For this review, take the finished solid that the model builds, in its own axes (mm). Face numbers are marked on the shaded views. A direction names the side the tool comes from. Coordinates: 2 decimals unless noted, no trailing zeros. Loops run counter-clockwise (first coordinate to the right, second up) from the corner with the lowest first, then second, coordinate; pieces in that order, holes last. Notation, with made-up numbers: (-13, 15) - (15, 15) arc R18 cw to (15, 45) - close; hole circle Ø7 at (31, 40). An arc over 180 degrees is marked (long way). One line per item, written item: value. Start each with the question number.
1. Take a section at A-A, the plane z = 10.75. State the section outline as (x, y) points, and give its area (3 significant figures).
2. To check wall thickness, follow line 1 (X direction, y = -37.5, z = 8.5); line 2 (Y direction, x = -3.5, z = 9.5); line 3 (Z direction, x = 22.5, y = -36). State the ranges of each line that lie inside material, in increasing order. Write a range as from..to.
3. Insertion check: pin 1 (6.5 mm diameter, centred on x = 11.5, y = -7.5, fed in from +Z); pin 2 (2.5 mm diameter, centred on x = -23.3, y = -35.37, fed in from +Z); pin 3 (2 mm diameter, centred on x = 16.5, z = 4.5, fed in from +Y). Each pin has a flat end and moves straight along its axis. Give the tip position at first contact, or say it passes through.
4. Take a section at B-B, the plane x = 4. State the section outline as (y, z) points.
5. Take a section at C-C, the plane y = -33. State the section outline as (x, z) points, and give its area (3 significant figures).
6. For the marked faces 1 and 2, list the 3-axis set-ups (+Z, -Z, +X, -X, +Y, -Y) from which the entire face can be reached by the end or side of a thin tool; tool diameter is ignored.
```python
from build123d import *

# Parameters (mm, degrees)
F0_W     = 65
F0_H     = 15
F0_R     = 2.85
F1_DEPTH = 12
F2_W     = 65
F2_H     = 13
F3_DEPTH = 8.8
F4_R     = 1.2
F5_R     = 1.05
F6_DEPTH = 15
F8_DEPTH = 6.9


with BuildPart() as f1:
    # F0 (on Top) → F1 (new body)
    with BuildSketch(Plane.XY):
        with Locations((0.397058, -10.369431)):
            Rectangle(F0_W, F0_H)
        with Locations((-20.602942, -9.369431)):
            Circle(F0_R, mode=Mode.SUBTRACT)
        with Locations((21.397058, -9.369431)):
            Circle(F0_R, mode=Mode.SUBTRACT)
        with BuildLine():
            Line((32.897058, -17.869431), (-32.102942, -17.869431))
            Line((-32.102942, -17.869431), (-32.102942, -35.869431))
            ThreePointArc((-32.102942, -35.869431), (-25.659291, -51.42578), (-10.102942, -57.869431))
            Line((-10.102942, -57.869431), (10.897058, -57.869431))
            ThreePointArc((10.897058, -57.869431), (26.453407, -51.42578), (32.897058, -35.869431))
            Line((32.897058, -35.869431), (32.897058, -17.869431))
        make_face()
    extrude(amount=F1_DEPTH)

    # F2 (on face) → F3 (cut)
    with BuildSketch(Plane.XY.offset(12)):
        with Locations((0.397058, -9.369431)):
            Rectangle(F2_W, F2_H)
    extrude(amount=-F3_DEPTH, mode=Mode.SUBTRACT)

    # F4
    f4_edges = [f1.edges().sort_by_distance(p)[0] for p in [
        (-32.102942, -19.369431, 0),
        (0.397058, -57.869431, 0),
        (32.897058, -19.369431, 0),
    ]]
    fillet(f4_edges, radius=F4_R)

    # F5 (on face) → F6 (cut)
    with BuildSketch(Plane(origin=(0, 0, 0), x_dir=(1, 0, 0), z_dir=(0, 0, -1))):
        with Locations((23.697058, 35.369431)):
            Circle(F5_R)
        with Locations((-23.302942, 35.369431)):
            Circle(F5_R)
    extrude(amount=-F6_DEPTH, mode=Mode.SUBTRACT)

    # F7 (on face) → F8 (cut)
    with BuildSketch(Plane.XY.offset(12)):
        Polygon((25.605654, -38.499621), (27.362181, -35.281633), (25.453585, -32.151443), (21.788462, -32.23924), (20.031935, -35.457228), (21.940531, -38.587419), align=None)
        Polygon((-21.394346, -38.499621), (-19.637819, -35.281633), (-21.546415, -32.151443), (-25.211538, -32.23924), (-26.968065, -35.457228), (-25.059469, -38.587419), align=None)
    extrude(amount=-F8_DEPTH, mode=Mode.SUBTRACT)


solid = f1.part
```
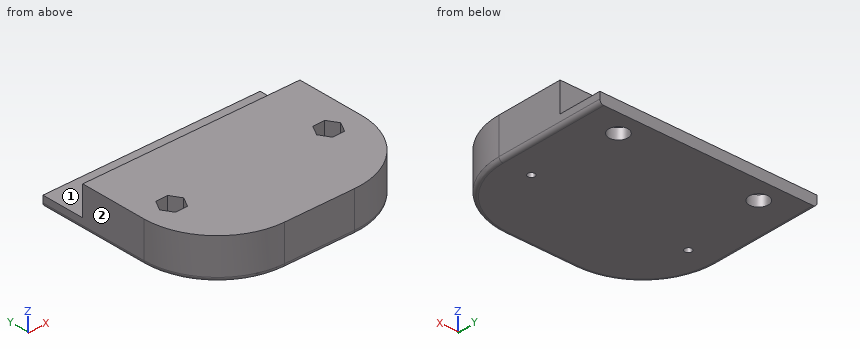
Solutions:
1. outline: (-32.1, -35.87) arc R22 ccw to (-10.1, -57.87) - (10.9, -57.87) arc R22 ccw to (32.9, -35.87) - (32.9, -15.87) - (-32.1, -15.87) - close; hole (-26.97, -35.46) - (-25.06, -38.59) - (-21.39, -38.5) - (-19.64, -35.28) - (-21.55, -32.15) - (-25.21, -32.24) - close; hole (20.03, -35.46) - (21.94, -38.59) - (25.61, -38.5) - (27.36, -35.28) - (25.45, -32.15) - (21.79, -32.24) - close
1. area: 2,450 mm2
2. line 1: -32.04..-25.72, -20.85..21.28, 26.15..32.84
2. line 2: -57.87..-15.87
2. line 3: 0..5.1
3. pin 1: z = 3.2
3. pin 2: z = 5.1
3. pin 3: y = -15.87
4. outline: (-57.87, 1.2) arc R1.2 ccw to (-56.67, 0) - (-2.87, 0) - (-2.87, 3.2) - (-15.87, 3.2) - (-15.87, 12) - (-57.87, 12) - close
5. outline: (-32.1, 1.2) arc R1.2 ccw to (-30.9, 0) - (31.7, 0) arc R1.2 ccw to (32.9, 1.2) - (32.9, 12) - (25.97, 12) - (25.97, 5.1) - (21.37, 5.1) - (21.37, 12) - (-21.03, 12) - (-21.03, 5.1) - (-25.63, 5.1) - (-25.63, 12) - (-32.1, 12) - close
5. area: 716 mm2
6. face 1: +Z, +X, -X, +Y
6. face 2: +Z, -Z, -X, +Y, -Y
